Autodesk Inventor part; units mm, degrees
ref_plane "Work Plane3" through (0, 0, 81) normal (0, 0, -1) x (-1, 0, 0)
ref_plane "Work Plane4" through (15, 0, 81) normal (1, 0, 0) x (0, 1, 0)
ref_plane "Work Plane5" through (0, 10, -53.2) normal (0, 1, 0) x (-1, 0, 0)
sketch "Sketch1" plane through (0, 0, 0) normal (0, 0, 1) x (1, 0, 0)
  circle A0 centre (0, 0) radius 10
  dimension "d0" = 20
extrude "Extrusion1" add sketch "Sketch1" along normal blind 65
sketch "Sketch2" plane through (0, 0, 65) normal (0, 0, 1) x (1, 0, 0)
  circle A0 centre (0, 0) radius 10
  dimension "d3" = 20
extrude "Extrusion2" add sketch "Sketch2" along normal blind 150
sketch "Sketch3" plane through (0, 0, 0) normal (0, 0, -1) x (-1, 0, 0)
  circle A0 centre (0, 0) radius 10
extrude "Extrusion3" add sketch "Sketch3" along normal blind 100
sketch "Sketch6" plane through (0, 0, -100) normal (0, 0, -1) x (-1, 0, 0)
  circle A0 centre (0, 0) radius 10
extrude "Extrusion4" cut sketch "Sketch6" against normal blind 54
sketch "Sketch7" plane through (0, 0, 215) normal (0, 0, 1) x (1, 0, 0)
  circle A0 centre (0, 0) radius 10
extrude "Extrusion5" add sketch "Sketch7" along normal blind 50
ref_plane "Work Plane3" through (0, 0, 81) normal (0, 0, -1) x (-1, 0, 0)
sketch "Sketch9" plane through (0, 0, 81) normal (0, 0, -1) x (-1, 0, 0)
  circle A0 centre (0, 0) radius 15
  dimension "d29" = 30
extrude "Extrusion7" add sketch "Sketch9" along normal blind 50
sketch "Sketch12" plane through (0, 0, -46) normal (0, 0, -1) x (-1, 0, 0)
  circle A0 centre (0, 0) radius 10
extrude "Extrusion8" add sketch "Sketch12" along normal blind 7.2
sketch "Sketch16" plane through (0, 0, 81) normal (0, 0, -1) x (-1, 0, 0)
  circle A0 centre (0, 0) radius 15
  point P0 (-15, 0)
ref_plane "Work Plane4" through (15, 0, 81) normal (1, 0, 0) x (0, 1, 0)
sketch "Sketch17" plane through (15, 0, 81) normal (1, 0, 0) x (0, 1, 0)
  line L0 (-15, -50) -> (15, -50)
  point P0 (0, -81)
  point P1 (0, -25)
  dimension "d67" = 25
hole "Hole4" at (15, 0, 56) direction (-1, 0, 0) diameter 4 end through all
sketch "Sketch18" plane through (0, 0, 265) normal (0, 0, 1) x (1, 0, 0)
  circle A0 centre (0, 0) radius 10
  line L0 (0, 10) -> (-2.5, 10)
  line L1 (-2.5, 10) -> (-2.5, 7.5)
  line L2 (-2.5, 7.5) -> (0, 7.5)
  line L3 (0, 10) -> (2.5, 10)
  line L4 (2.5, 10) -> (2.5, 7.5)
  line L5 (2.5, 7.5) -> (0, 7.5)
  point P0 (0, 7.5)
  point P1 (2.5, 9.6825)
  point P2 (-2.5, 9.6825)
  dimension "d75" = 5
  dimension "d76" = 2.5
  dimension "d77" = 10
extrude "Extrusion12" cut sketch "Sketch18" against normal blind 30 contours L4 L5 L2 L1 A0 picked at (1.3922, 8.2862)
sketch "Sketch19" plane through (0, 0, -53.2) normal (0, 0, -1) x (-1, 0, 0)
  circle A0 centre (0, 0) radius 3
  dimension "d80" = 6
extrude "Extrusion13" cut sketch "Sketch19" against normal blind 13
sketch "Sketch20" plane through (0, 0, -53.2) normal (0, 0, -1) x (-1, 0, 0)
  point P0 (0, 0)
  point P1 (0, 10)
ref_plane "Work Plane5" through (0, 10, -53.2) normal (0, 1, 0) x (-1, 0, 0)
sketch "Sketch21" plane through (0, 10, -53.2) normal (0, 1, 0) x (-1, 0, 0)
  line L0 (-10, 0) -> (10, 0)
  point P0 (0, 53.2)
  point P1 (0, 6.5)
  dimension "d83" = 6.5
hole "Hole5" at (0, 10, -46.7) direction (0, -1, 0) diameter 3.242 depth 9 tip angle 118
equation "\"d73\" = Thickness"
equation "\"BendRadius\" = Thickness"
equation "\"BendReliefWidth\" = Thickness"
equation "\"BendReliefDepth\" = 0.5 * Thickness"
equation "\"CornerReliefSize\" = 4 * Thickness"
equation "\"MinimumRemnant\" = 2 * Thickness"
equation "\"TransitionRadius\" = BendRadius"
equation "\"JacobiRadiusSize\" = BendRadius"
equation "\"GapSize\" = Thickness"
properties part number "Rough draft shaft"
Input: part model. Units: mm. Frame: model coordinates. A direction names the side the tool comes from. Give positions to 0.01 mm unless a question says otherwise; leave off trailing zeros. Loops run counter-clockwise (first coordinate to the right, second up) from the corner with the lowest first, then second, coordinate; pieces in that order, holes last. Notation, with made-up numbers: M 64,85 L 72,85 A29 ccw 72,109 Z; hole C 39.5,10 d5. An arc over 180 degrees is marked long. Use CSV: the item, a comma, the result in double quotes.
(1) Pin query (flat end, axial travel): P1, Ø6, axis at x = -4.5, z = 200, coming from the -Y side; P2, Ø15, axis at x = 1, y = 2, coming from the -Z side; P3, Ø3, axis at x = 0, z = -46.7, coming from the -Y side; P4, Ø2.5, axis at y = 8.5, z = 245, coming from the -X side. Return the tip coordinate at first contact, or that it passes through.
Outcome:
P1,"stops at y = -9.89"
P2,"stops at z = -53.2"
P3,"stops at y = -10"
P4,"stops at x = -6.89"
(2) Set-up query: faces 1 (the face through (-3, -10, 31)), 2 (the face through (0, 0, 265)), 3 (the face through (0, 7.5, 250)). Return all of +Z, -Z, +X, -X, +Y, -Y with unobstructed straight access to the full face (end or side cutting, diameter ignored); none if empty.
Outcome:
face 1,"-Z"
face 2,"+Z, +X, -X, +Y, -Y"
face 3,"+Z, +Y"
(3) Section A-A, the plane x = 6.5. Return loops of the section in (y, z), plus the area to 3 significant figures.
Outcome:
outline,"M -13.52,31 L -7.6,31 L -7.6,-53.2 L 7.6,-53.2 L 7.6,31 L 13.52,31 L 13.52,81 L 7.6,81 L 7.6,265 L -7.6,265 L -7.6,81 L -13.52,81 Z; hole C 0,56 d4"
area,"5,420 mm²"
(4) Pull-direction query (Y, two-part tool) for faces 4 (the face through (5.38, -8.43, 171.71)), 5 (the face through (-3, -10, 81)), 6 (the face through (0.65, -2.93, -46.79)); classes: pulls with the +Y half, pulls with the -Y half, needs draft (parallel to the pull), parting line crosses it, or undercut.
Outcome:
face 4,"parting line crosses it"
face 5,"needs draft"
face 6,"undercut"
(5) Material intervals for L1, parallel to Y at x = 1, z = 56; L2, parallel to Z at x = -9, y = 5; L3, parallel to Y at x = 0, z = -48, sorted ascending. Write a range as [from, to].
Outcome:
L1,"y = [-14.97, -2], [2, 14.97]"
L2,"z = [31, 81]"
L3,"y = [-10, -3]"
(6) Section B-B, the plane y = -6. Return loops of the section in (x, z), plus the area to 3 significant figures.
Outcome:
outline,"M -13.75,31 L -8,31 L -8,-53.2 L 8,-53.2 L 8,31 L 13.75,31 L 13.75,81 L 8,81 L 8,265 L -8,265 L -8,81 L -13.75,81 Z"
area,"5,670 mm²"
(7) Section D-D, the plane x = -6. Return loops of the section in (y, z).
Outcome:
outline,"M -13.75,31 L -8,31 L -8,-53.2 L 8,-53.2 L 8,31 L 13.75,31 L 13.75,81 L 8,81 L 8,265 L -8,265 L -8,81 L -13.75,81 Z; hole C 0,56 d4"
(8) Section C-C, the plane z = 115. Return loops of the section in (x, y), plus the area to 3 significant figures.
Outcome:
outline,"C 0,0 d20"
area,"314 mm²"
